Work out the finished part from the listing and answer in its coordinate system (mm). A direction names the side the tool comes from. Round coordinates to 2 decimals unless told otherwise and drop trailing zeros. Write each loop counter-clockwise with the first axis right and the second up, starting at its lowest first coordinate (ties: lowest second). Pieces come first, ordered by that corner, then holes. Notation, with made-up numbers: (41, -12.5) - (89, -12.5) arc R24 cw to (89, -2.5) - close; hole circle Ø1 at (24, 15). An arc over 180 degrees is marked (long way). Answer as a JSON object with one key per item and string values.
```python
from build123d import *

# Parameters (mm, degrees)
F1_DEPTH = 50
F2_W     = 30
F2_H     = 18.285982
F3_DEPTH = 92.000995


with BuildPart() as f1:
    # F0 (on Front) → F1 (new body)
    with BuildSketch(Plane.XZ):
        Polygon((0, 15.090908), (0, 0), (40.363642, 0), (40.363642, 10), (12.363637, 10), (12.363637, 50), (-7.636363, 50), (-7.636363, 40.545456), (-32.363635, 40.545456), (-32.363635, 50), (-52.363635, 50), (-52.363635, 10), (-79.636358, 10), (-79.636358, 0), (-40, 0), (-40, 15.090908), align=None)
    extrude(amount=-F1_DEPTH)

    # F2 (on face) → F3 (cut, through all)
    with BuildSketch(Plane.YZ.offset(12.363637)):
        with Locations((25, 40.857009)):
            Rectangle(F2_W, F2_H)
    extrude(amount=-F3_DEPTH, mode=Mode.SUBTRACT)


solid = f1.part
```
Item 1: Consider line 1 along X through (y, z) = (26, 11); line 2 along X through (y, z) = (5, 9.5); line 3 along Z through (x, y) = (-19, 45.5). Determine where each line is inside the solid, lowest interval first.
Results found:
{"line 1": "-52.36 to -40, 0 to 12.36", "line 2": "-79.64 to -40, 0 to 40.36", "line 3": "15.09 to 40.55"}
Item 2: Determine the mould class of faces 1 (the flat face through (40.364, 25, 5)), 2 (the flat face through (-20, 5, 40.545)), 3 (the flat face through (27, 25, 10)) for opening direction X: pulls with the +X half, pulls with the -X half, needs draft (parallel to the pull), parting line crosses it, or undercut.
Results found:
{"face 1": "pulls with the +X half", "face 2": "undercut", "face 3": "needs draft"}
Item 3: A cutting plane is placed at C-C (y = 45). Write down the section's boundary in (x, z).
Results found:
{"outline": "(-79.64, 0) - (-40, 0) - (-40, 15.09) - (0, 15.09) - (0, 0) - (40.36, 0) - (40.36, 10) - (12.36, 10) - (12.36, 50) - (-7.64, 50) - (-7.64, 40.55) - (-32.36, 40.55) - (-32.36, 50) - (-52.36, 50) - (-52.36, 10) - (-79.64, 10) - close"}
Item 4: For faces 4 (the flat face through (12.364, 25, 25)), 5 (the flat face through (-20, 40, 39)), 6 (the flat face through (0, 25, 8)), 7 (the flat face through (-32.364, 45, 45)), determine the directions among +Z, -Z, +X, -X, +Y, -Y from which every point of the face is accessible in a straight line to the end or side of a thin tool.
Results found:
{"face 4": "+Z, +X, +Y, -Y", "face 5": "+Z, +X, -X", "face 6": "-Z, +Y, -Y", "face 7": "+Z, +Y, -Y"}
Item 5: A cutting plane is placed at B-B (z = 6). Write down the section's boundary in (x, y), and give its area (3 significant figures).
Results found:
{"outline": "(-79.64, 0) - (-40, 0) - (-40, 50) - (-79.64, 50) - close; (0, 0) - (40.36, 0) - (40.36, 50) - (0, 50) - close", "area": "4,000 mm²"}
Item 6: A cutting plane is placed at A-A (x = -48). Write down the section's boundary in (y, z).
Results found:
{"outline": "(0, 0) - (50, 0) - (50, 50) - (40, 50) - (40, 31.71) - (10, 31.71) - (10, 50) - (0, 50) - close"}
Item 7: A cutting plane is placed at D-D (z = 34.5). Write down the section's boundary in (x, y), and give its area (3 significant figures).
Results found:
{"outline": "(-52.36, 0) - (12.36, 0) - (12.36, 10) - (-52.36, 10) - close; (-52.36, 40) - (12.36, 40) - (12.36, 50) - (-52.36, 50) - close", "area": "1,290 mm²"}
Item 8: Each of these flat-tipped pins is pushed along its axis until it touches: P1, Ø24, axis at x = -6, y = 25, coming from the +Z side; P2, Ø3, axis at y = 47, z = 47.5, coming from the -X side; P3, Ø4.5, axis at y = 45, z = 46, coming from the +X side. Where does it stop, or does it pass through?
Results found:
{"P1": "z = 31.71", "P2": "x = -52.36", "P3": "x = 12.36"}
